Could you check a few things on this model? Use its own coordinates, in mm. Round coordinates to 2 decimals unless told otherwise and drop trailing zeros. Order: outer loops, then holes, each group sorted by start corner. A loop starts at its lowest first (then second) coordinate and runs counter-clockwise, first axis right, second up. Notation, with made-up numbers: M 20.25,-28 L 76.25,-28 A34 ccw 76.25,2 Z; hole C 43,24 d7. An arc over 180 degrees is marked long. Write each question's results on one line, items separated by ' | '. Start each with the question number.
1. We'd pull the mould along Z, two halves only. Please class faces 1 (the cylindrical face through (1.01, 68.89, -19.1)), 2 (the cylindrical face through (0.986, 47.345, 0.867)), 3 (the cylindrical face through (1.01, 68.85, 19.14)): released by +Z, released by -Z, zero draft, split by the parting line, or undercut.
2. Suppose I cut it at C-C on y = -17.75. Write out the boundary of the cut face in (x, z), and give its area (3 significant figures).
3. Please list where these lines run through material, in increasing order: L1, parallel to Y at x = 1.4, z = -7.5; L2, parallel to Y at x = 0.2, z = 1; L3, parallel to Z at x = 1.95, y = 29.
4. Suppose I cut it at A-A on z = 12.5. Write out the boundary of the cut face in (x, y).
5. Suppose I cut it at D-D on x = 1.6. Give the number of separate pieces and of enclosed holes in the cut face, and give its area (3 significant figures).
6. Suppose I cut it at B-B on y = 51.25. Write out the boundary of the cut face in (x, z), and give its area (3 significant figures).
7. I'm going to push flat-ended pins straight in: pin 1 (1 mm diameter, centred on x = 2, z = 15, fed in from +Y); pin 2 (1 mm diameter, centred on x = 0.5, y = -56, fed in from +Z); pin 3 (1 mm diameter, centred on x = 1, z = 21, fed in from +Y). Where does each tip first touch, or does it pass through?
from build123d import *

# Parameters (mm, degrees)
SKETCH_1_W      = 40
SKETCH_1_H      = 139.5
SKETCH_1_R      = 7
SKETCH_1_R_2    = 1.6
SKETCH_1_R_3    = 4
SKETCH_1_W_2    = 20
SKETCH_1_H_2    = 12
SKETCH_1_W_3    = 3
SKETCH_1_H_3    = 50
EXTRUDE_1_DEPTH = 2
FILLET_1_R      = 3
FILLET_2_R      = 1


with BuildPart() as part:
    # 草图1 → 凸台-拉伸1 (new body)
    # profile 1 of 4: a face of its own
    with BuildSketch(Plane(origin=(0, 0, 0), x_dir=(0, 0, -1), z_dir=(1, 0, 0))):
        Rectangle(SKETCH_1_W, SKETCH_1_H)
        with Locations((0, -17.75)):
            Circle(SKETCH_1_R, mode=Mode.SUBTRACT)
        with Locations((0, -5.25)):
            Circle(SKETCH_1_R_2, mode=Mode.SUBTRACT)
        with Locations((12.5, -17.75)):
            Circle(SKETCH_1_R_2, mode=Mode.SUBTRACT)
        with Locations((0, -30.25)):
            Circle(SKETCH_1_R_2, mode=Mode.SUBTRACT)
        with Locations((-12.5, -17.75)):
            Circle(SKETCH_1_R_2, mode=Mode.SUBTRACT)
        with Locations((-6.5, 15.25)):
            Circle(SKETCH_1_R_2, mode=Mode.SUBTRACT)
        with Locations((6.5, 15.25)):
            Circle(SKETCH_1_R_2, mode=Mode.SUBTRACT)
        with Locations((0, 51.25)):
            Circle(SKETCH_1_R_3, mode=Mode.SUBTRACT)
    # profile 2 of 4: a face of its own
    with BuildSketch(Plane(origin=(0, 0, 0), x_dir=(0, 0, -1), z_dir=(1, 0, 0))):
        with Locations((0, 75.75)):
            Rectangle(SKETCH_1_W_2, SKETCH_1_H_2)
        with Locations((-6.5, 78.25)):
            Circle(SKETCH_1_R_2, mode=Mode.SUBTRACT)
        with Locations((6.5, 78.25)):
            Circle(SKETCH_1_R_2, mode=Mode.SUBTRACT)
    # profile 3 of 4: a face of its own
    with BuildSketch(Plane(origin=(0, 0, 0), x_dir=(0, 0, -1), z_dir=(1, 0, 0))):
        with Locations((21.5, -12.75)):
            Rectangle(SKETCH_1_W_3, SKETCH_1_H_3)
    # profile 4 of 4: a face of its own
    with BuildSketch(Plane(origin=(0, 0, 0), x_dir=(0, 0, -1), z_dir=(1, 0, 0))):
        with Locations((-21.5, -12.75)):
            Rectangle(SKETCH_1_W_3, SKETCH_1_H_3)
    extrude(amount=EXTRUDE_1_DEPTH)

    # 圆角1
    fillet_1_edges = [part.edges().sort_by_distance(p)[0] for p in [
        (1, 69.75, 20),
        (1, 81.75, 10),
        (1, 81.75, -10),
        (1, 69.75, -20),
    ]]
    fillet(fillet_1_edges, radius=FILLET_1_R)

    # 圆角2
    fillet_2_edges = [part.edges().sort_by_distance(p)[0] for p in [
        (1, -69.75, 20),
        (1, -37.75, 23),
        (1, 12.25, 23),
        (1, 12.25, -23),
        (1, -37.75, -23),
        (1, -69.75, -20),
    ]]
    fillet(fillet_2_edges, radius=FILLET_2_R)


solid = part.part
Filled sheet:
1) face 1: released by -Z | face 2: undercut | face 3: released by +Z
2) outline: M 0,-23 L 2,-23 L 2,-14.1 L 0,-14.1 Z; M 0,-10.9 L 2,-10.9 L 2,-7 L 0,-7 Z; M 0,7 L 2,7 L 2,10.9 L 0,10.9 Z; M 0,14.1 L 2,14.1 L 2,23 L 0,23 Z | area: 51.2 mm^2
3) L1: y = -69.75 to 14, 16.5 to 77, 79.5 to 81.71 | L2: y = -69.75 to -31.5, -29 to -24.68, -10.82 to -6.5, -4 to 47.38, 55.12 to 81.75 | L3: z = -20 to 20
4) outline: M 0,-69.75 L 2,-69.75 L 2,-19.35 L 0,-19.35 Z; M 0,-16.15 L 2,-16.15 L 2,69.75 L 0,69.75 Z
5) separate pieces: 1 | enclosed holes: 10 | area: 5,840 mm^2
6) outline: M 0,-20 L 2,-20 L 2,-4 L 0,-4 Z; M 0,4 L 2,4 L 2,20 L 0,20 Z | area: 64.0 mm^2
7) pin 1: stops at y = 69.75 | pin 2: stops at z = 20 | pin 3: stops at y = 12.25
